Read the model definition and answer for the solid it produces. Units are mm, in the model's axes. A direction names the side the tool comes from. Coordinates: 2 decimals unless noted, no trailing zeros. Write each loop counter-clockwise with the first axis right and the second up, starting at its lowest first coordinate (ties: lowest second). Pieces come first, ordered by that corner, then holes.
(1) Given pin 1 (10 mm diameter, centred on x = 22.5, z = 0.5, fed in from -Y); pin 2 (4 mm diameter, centred on y = -7.5, z = 16.5, fed in from -X), each flat-ended and moving along its own axis, determine where each tip first touches the part or whether it passes through.
(2) Section B-B on x = 13 is taken. Write down the section's boundary in (y, z), then the cut area to 3 significant figures.
(3) Section C-C on z = -5 is taken. Write down the section's boundary in (x, y), then the cut area to 3 significant figures.
(4) Find the intervals of material crossed by probe 1 along Z at (x, y) = (-8, 1.7); probe 2 along Z at (x, y) = (4, -5.5); probe 3 along Y at (x, z) = (29.45, 18), in increasing order.
(5) The mould has two halves that part along Z. Classify faces 1 (the flat face through (15, -3, -27.5)), 2 (the cylindrical face through (-8.488, 2.465, 17.804)), 3 (the flat face through (15, -3, 27.5)): +Z half, -Z half, draft (parallel to the pull), parting line (faces both ways), or undercut.
(6) Section A-A on y = -9 is taken. Write down the section's boundary in (x, z), then the cut area to 3 significant figures.
(7) Section D-D on x = -0.5 is taken. Write down the section's boundary in (y, z), then the cut area to 3 significant figures.
(8) Which of the six approach directions +Z, -Z, +X, -X, +Y, -Y give full straight-line access (tool end or side, diameter ignored) to faces 4 (the flat face through (12, -6, -24.5)), 5 (the cylindrical face through (30.5, -7.4, -15.5))?
from build123d import *

# Parameters (mm, degrees)
SKETCH1_W           = 30
SKETCH1_H           = 55
BOSS_EXTRUDE1_DEPTH = 5
SKETCH4_W           = 55
SKETCH4_H           = 5
BOSS_EXTRUDE2_DEPTH = 18
SKETCH5_W           = 55
SKETCH5_H           = 20
BOSS_EXTRUDE3_DEPTH = 5
SKETCH6_R           = 2.5
CUT_EXTRUDE3_DEPTH  = 5
BOSS_EXTRUDE4_DEPTH = 3
SKETCH8_R           = 2.25
CUT_EXTRUDE4_DEPTH  = 10


with BuildPart() as part:
    # Sketch1 → Boss-Extrude1 (new body)
    with BuildSketch(Plane(origin=(0, 0, 0), x_dir=(1, 0, 0), z_dir=(0, 1, 0))):
        Rectangle(SKETCH1_W, SKETCH1_H)
    extrude(amount=BOSS_EXTRUDE1_DEPTH)

    # Sketch4 → Boss-Extrude2 (add)
    with BuildSketch(Plane(origin=(15, 0, 0), x_dir=(0, 0, -1), z_dir=(1, 0, 0))):
        with Locations((0, 2.5)):
            Rectangle(SKETCH4_W, SKETCH4_H)
    extrude(amount=BOSS_EXTRUDE2_DEPTH)

    # Sketch5 → Boss-Extrude3 (add)
    with BuildSketch(Plane(origin=(33, 0, 0), x_dir=(0, 0, -1), z_dir=(1, 0, 0))):
        with Locations((0, -5)):
            Rectangle(SKETCH5_W, SKETCH5_H)
    extrude(amount=-BOSS_EXTRUDE3_DEPTH)

    # Sketch6 → Cut-Extrude3 (cut)
    with BuildSketch(Plane(origin=(33, 0, 0), x_dir=(0, 0, -1), z_dir=(1, 0, 0))):
        with Locations((18, -7.5)):
            Circle(SKETCH6_R)
        with Locations((-18, -7.5)):
            Circle(SKETCH6_R)
    extrude(amount=-CUT_EXTRUDE3_DEPTH, mode=Mode.SUBTRACT)

    # Sketch7 → Boss-Extrude4 (add)
    with BuildSketch(Plane.XY.offset(27.5)):
        Polygon((28, -15), (-15, 0), (28, 0), align=None)
    boss_extrude4 = extrude(amount=-BOSS_EXTRUDE4_DEPTH)

    # Mirror1: Boss-Extrude4 across plane
    add(boss_extrude4.mirror(Plane.XY))

    # Sketch8 → Cut-Extrude4 (cut)
    with BuildSketch(Plane.XZ):
        with Locations((-8, 20)):
            Circle(SKETCH8_R)
        with Locations((-8, -20)):
            Circle(SKETCH8_R)
        with Locations((12, 20)):
            Circle(SKETCH8_R)
        with Locations((12, -20)):
            Circle(SKETCH8_R)
    extrude(amount=-CUT_EXTRUDE4_DEPTH, mode=Mode.SUBTRACT)


solid = part.part
Response:
1. pin 1: stops at y = 0
1. pin 2: stops at x = 28
2. outline: (-9.77, -27.5) - (5, -27.5) - (5, -22.02) - (0, -22.02) - (0, -24.5) - (-9.77, -24.5) - close; (-9.77, 24.5) - (0, 24.5) - (0, 22.02) - (5, 22.02) - (5, 27.5) - (-9.77, 27.5) - close; (0, -17.98) - (5, -17.98) - (5, 17.98) - (0, 17.98) - close
2. area: 293 mm2
3. outline: (-15, 0) - (28, 0) - (28, -15) - (33, -15) - (33, 5) - (-15, 5) - close
3. area: 315 mm2
4. probe 1: z = -27.5 to -22.25, -17.75 to 17.75, 22.25 to 27.5
4. probe 2: z = -27.5 to -24.5, 24.5 to 27.5
4. probe 3: y = -15 to -10, -5 to 5
5. face 1: -Z half
5. face 2: undercut
5. face 3: +Z half
6. outline: (10.8, -27.5) - (33, -27.5) - (33, -20) - (28, -20) - (28, -24.5) - (10.8, -24.5) - close; (10.8, 24.5) - (28, 24.5) - (28, 20) - (33, 20) - (33, 27.5) - (10.8, 27.5) - close; (28, -16) - (33, -16) - (33, 16) - (28, 16) - close
6. area: 338 mm2
7. outline: (-5.06, -27.5) - (5, -27.5) - (5, 27.5) - (-5.06, 27.5) - (-5.06, 24.5) - (0, 24.5) - (0, -24.5) - (-5.06, -24.5) - close
7. area: 305 mm2
8. face 4: -X, -Y
8. face 5: +X, -X
